from build123d import *

# Parameters (mm, degrees)
SKETCH_1_R          = 20
EXTRUDE_1_DEPTH     = 12
HOLE_WIZARD_M12_1_D = 10.2


with BuildPart() as part:
    # 草图1 → 凸台-拉伸1 (new body)
    with BuildSketch(Plane(origin=(0, 0, 0), x_dir=(0, 0, -1), z_dir=(1, 0, 0))):
        with BuildLine():
            Line((-40, 0), (-40, 70))
            Line((-40, 70), (40, 70))
            Line((40, 70), (40, 0))
            ThreePointArc((40, 0), (0, -40), (-40, 0))
        make_face()
        Circle(SKETCH_1_R, mode=Mode.SUBTRACT)
    extrude(amount=EXTRUDE_1_DEPTH)

    # M12 螺纹孔1 (through all)
    with Locations(Plane(origin=(12, 0, 0), x_dir=(0, 0, -1), z_dir=(1, 0, 0))):
        with Locations((0, 40)):
            Hole(HOLE_WIZARD_M12_1_D / 2)


solid = part.part
Geometry check sheet. Reference: the model listing, model coordinates, mm. Round coordinates to 2 decimals unless told otherwise and drop trailing zeros. Order: outer loops, then holes, each group sorted by start corner. A loop starts at its lowest first (then second) coordinate and runs counter-clockwise, first axis right, second up. Notation, with made-up numbers: M 52,11.5 L 60,11.5 A21 ccw 60,16.5 Z; hole C 59.5,26.25 d7. An arc over 180 degrees is marked long. Answer in a Markdown table with one row per item.
(1) Sectioned sample at C-C, the plane x = 5.75. Record the cut outline in (y, z), and give its area (3 significant figures).
Responses:
| item | result |
|---|---|
| outline | M 0,-40 L 70,-40 L 70,40 L 0,40 A40 ccw Z; hole C 0,0 d40; hole C 40,0 d10.2 |
| area | 6,770 mm² |
(2) Sectioned sample at A-A, the plane z = 0. Record the cut outline in (x, y).
Responses:
| item | result |
|---|---|
| outline | M 0,-40 L 12,-40 L 12,-20 L 0,-20 Z; M 0,20 L 12,20 L 12,34.9 L 0,34.9 Z; M 0,45.1 L 12,45.1 L 12,70 L 0,70 Z |
(3) Sectioned sample at B-B, the plane y = -14. Record the cut outline in (x, z).
Responses:
| item | result |
|---|---|
| outline | M 0,-37.47 L 12,-37.47 L 12,-14.28 L 0,-14.28 Z; M 0,14.28 L 12,14.28 L 12,37.47 L 0,37.47 Z |
(4) Go/stop test with flat-tipped pins: P1, Ø3, axis at x = 5.5, y = -7, coming from the +Z side; P2, Ø3, axis at y = -15, z = -16, coming from the -X side; P3, Ø6, axis at x = 8.5, z = 10.5, coming from the -Y side; P4, Ø2, axis at x = 3, y = -2, coming from the +Z side. Record where each tip stops, or that it passes through.
Responses:
| item | result |
|---|---|
| P1 | stops at z = 39.62 |
| P2 | stops at x = 0 |
| P3 | stops at y = -39.29 |
| P4 | stops at z = 39.99 |
(5) Sectioned sample at D-D, the plane z = -18.5. Record the cut outline in (x, y).
Responses:
| item | result |
|---|---|
| outline | M 0,-35.46 L 12,-35.46 L 12,-7.6 L 0,-7.6 Z; M 0,7.6 L 12,7.6 L 12,70 L 0,70 Z |
(6) Draft check along Z on faces 1 (the face through (5.9, 35.5, 2.4)), 2 (the face through (6, 35, -40)), 3 (the face through (6, 70, 1)). Enter one of: released by +Z, released by -Z, zero draft, split by the parting line, or undercut.
Responses:
| item | result |
|---|---|
| face 1 | undercut |
| face 2 | released by -Z |
| face 3 | zero draft |
(7) Scan lines: probe 1 along Y at (x, z) = (4.25, 0); probe 2 along Y at (x, z) = (4.75, -1); probe 3 along Z at (x, y) = (1.5, -3). Record each from-to range of solid material in increasing order. Write a range as from..to.
Responses:
| item | result |
|---|---|
| probe 1 | y = -40..-20, 20..34.9, 45.1..70 |
| probe 2 | y = -39.99..-19.97, 19.97..35, 45..70 |
| probe 3 | z = -39.89..-19.77, 19.77..39.89 |
